Read the model definition and answer for the solid it produces. Units are mm, in the model's axes. Face numbers are marked on the shaded views. A direction names the side the tool comes from. Coordinates: 2 decimals unless noted, no trailing zeros. Write each loop counter-clockwise with the first axis right and the second up, starting at its lowest first coordinate (ties: lowest second). Pieces come first, ordered by that corner, then holes.
(1) Section B-B on y = 6.25 is taken. State how many separate pieces and enclosed holes the cut face has, then the cut area to 3 significant figures.
(2) Which of the six approach directions +Z, -Z, +X, -X, +Y, -Y give full straight-line access (tool end or side, diameter ignored) to the marked faces 4 and 5?
(3) Section A-A on x = 0 is taken. Write down the section's boundary in (y, z) (3 decimals), then the cut area to 3 significant figures.
(4) Given pin 1 (4 mm diameter, centred on x = -14, y = 3, fed in from -Z); pin 2 (6.5 mm diameter, centred on y = -1, z = 35, fed in from -X); pin 3 (11 mm diameter, centred on x = -43, y = -5, fed in from -Z); pin 4 (12 mm diameter, centred on x = -14, z = 55, fed in from +Y), each flat-ended and moving along its own axis, determine where each tip first touches the part or whether it passes through.
(5) Find the intervals of material crossed by probe 1 along Z at (x, y) = (-25.5, -3.5); probe 2 along X at (y, z) = (11.25, -43); probe 3 along X at (y, z) = (-9.75, -43), in increasing order.
(6) The mould has two halves that part along X. Classify the marked faces 1, 2 and 3: +X half, -X half, draft (parallel to the pull), parting line (faces both ways), or undercut.
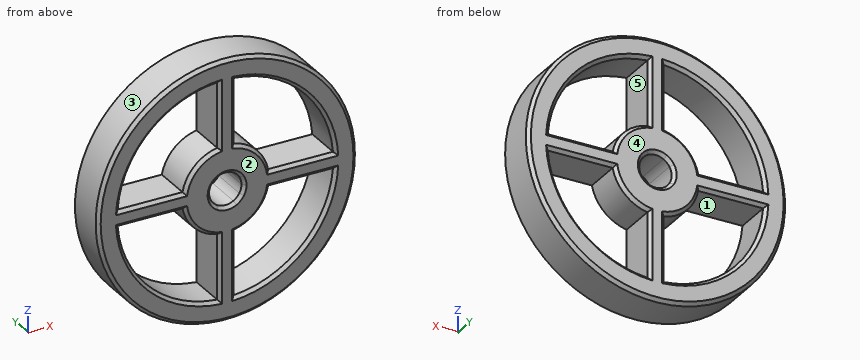
from build123d import *

# Parameters (mm, degrees)
F0_R     = 76.2
F1_DEPTH = 12.7
F2_SIZE  = 1.905
F3_SIZE  = 1.905


with BuildPart() as f1:
    # F0 (on Front) → F1 (new body, symmetric)
    with BuildSketch(Plane.XZ):
        Circle(F0_R)
        with BuildLine():
            ThreePointArc((-4.7625, -63.321154), (-44.901281, -44.901281), (-63.321154, -4.7625))
            Line((-63.321154, -4.7625), (-25.160792, -4.7625))
            Line((-25.160792, -4.7625), (-8.248892, -4.7625))
            ThreePointArc((-8.248892, -4.7625), (-9.525, 0), (-8.248892, 4.7625))
            Line((-8.248892, 4.7625), (-25.160792, 4.7625))
            Line((-25.160792, 4.7625), (-63.321154, 4.7625))
            ThreePointArc((-63.321154, 4.7625), (-44.901281, 44.901281), (-4.7625, 63.321154))
            Line((-4.7625, 63.321154), (-4.7625, 25.160792))
            Line((-4.7625, 25.160792), (-4.7625, 8.248892))
            ThreePointArc((-4.7625, 8.248892), (0, 9.525), (4.7625, 8.248892))
            Line((4.7625, 8.248892), (4.7625, 25.160792))
            Line((4.7625, 25.160792), (4.7625, 63.321154))
            ThreePointArc((4.7625, 63.321154), (44.901281, 44.901281), (63.321154, 4.7625))
            Line((63.321154, 4.7625), (25.160792, 4.7625))
            Line((25.160792, 4.7625), (8.248892, 4.7625))
            ThreePointArc((8.248892, 4.7625), (9.200443, 2.465251), (9.525, 0))
            ThreePointArc((9.525, 0), (9.200443, -2.465251), (8.248892, -4.7625))
            Line((8.248892, -4.7625), (25.160792, -4.7625))
            Line((25.160792, -4.7625), (63.321154, -4.7625))
            ThreePointArc((63.321154, -4.7625), (44.901281, -44.901281), (4.7625, -63.321154))
            Line((4.7625, -63.321154), (4.7625, -25.160792))
            Line((4.7625, -25.160792), (4.7625, -8.248892))
            ThreePointArc((4.7625, -8.248892), (0, -9.525), (-4.7625, -8.248892))
            Line((-4.7625, -8.248892), (-4.7625, -25.160792))
            Line((-4.7625, -25.160792), (-4.7625, -63.321154))
        make_face(mode=Mode.SUBTRACT)
        with BuildLine():
            Line((-25.160792, 4.7625), (-8.248892, 4.7625))
            ThreePointArc((-8.248892, 4.7625), (-6.735192, 6.735192), (-4.7625, 8.248892))
            Line((-4.7625, 8.248892), (-4.7625, 25.160792))
            ThreePointArc((-4.7625, 25.160792), (-18.107275, 18.107275), (-25.160792, 4.7625))
        make_face()
        with BuildLine():
            Line((4.7625, 25.160792), (4.7625, 8.248892))
            ThreePointArc((4.7625, 8.248892), (6.735192, 6.735192), (8.248892, 4.7625))
            Line((8.248892, 4.7625), (25.160792, 4.7625))
            ThreePointArc((25.160792, 4.7625), (18.107275, 18.107275), (4.7625, 25.160792))
        make_face()
        with BuildLine():
            ThreePointArc((8.248892, -4.7625), (6.735192, -6.735192), (4.7625, -8.248892))
            Line((4.7625, -8.248892), (4.7625, -25.160792))
            ThreePointArc((4.7625, -25.160792), (18.107275, -18.107275), (25.160792, -4.7625))
            Line((25.160792, -4.7625), (8.248892, -4.7625))
        make_face()
        with BuildLine():
            Line((-8.248892, -4.7625), (-25.160792, -4.7625))
            ThreePointArc((-25.160792, -4.7625), (-18.107275, -18.107275), (-4.7625, -25.160792))
            Line((-4.7625, -25.160792), (-4.7625, -8.248892))
            ThreePointArc((-4.7625, -8.248892), (-6.735192, -6.735192), (-8.248892, -4.7625))
        make_face()
    extrude(amount=F1_DEPTH, both=True)

    # F2
    f2_edges = [f1.edges().sort_by_distance(p)[0] for p in [
        (-76.2, -12.7, 0),
        (-4.7625, -12.7, -44.240973),
        (-44.901281, -12.7, -44.901281),
        (-44.240973, -12.7, -4.7625),
        (-18.107275, -12.7, -18.107275),
        (4.7625, -12.7, 8.248892),
        (44.240973, -12.7, -4.7625),
        (44.901281, -12.7, -44.901281),
        (4.7625, -12.7, -44.240973),
        (18.107275, -12.7, -18.107275),
        (4.7625, -12.7, 44.240973),
        (44.901281, -12.7, 44.901281),
        (44.240973, -12.7, 4.7625),
        (18.107275, -12.7, 18.107275),
        (-44.240973, -12.7, 4.7625),
        (-44.901281, -12.7, 44.901281),
        (-4.7625, -12.7, 44.240973),
        (-18.107275, -12.7, 18.107275),
    ]]
    chamfer(f2_edges, length=F2_SIZE)

    # F3
    f3_edges = [f1.edges().sort_by_distance(p)[0] for p in [
        (-76.2, 12.7, 0),
        (4.7625, 12.7, 8.248892),
        (-4.7625, 12.7, -44.240973),
        (-44.901281, 12.7, -44.901281),
        (-44.240973, 12.7, -4.7625),
        (-18.107275, 12.7, -18.107275),
        (44.240973, 12.7, -4.7625),
        (44.901281, 12.7, -44.901281),
        (4.7625, 12.7, -44.240973),
        (18.107275, 12.7, -18.107275),
        (4.7625, 12.7, 44.240973),
        (44.901281, 12.7, 44.901281),
        (44.240973, 12.7, 4.7625),
        (18.107275, 12.7, 18.107275),
        (-44.240973, 12.7, 4.7625),
        (-44.901281, 12.7, 44.901281),
        (-4.7625, 12.7, 44.240973),
        (-18.107275, 12.7, 18.107275),
    ]]
    chamfer(f3_edges, length=F3_SIZE)


solid = f1.part
Response:
1. separate pieces: 1
1. enclosed holes: 5
1. area: 8,800 mm2
2. face 4: +Z, -Z, +X, -X, +Y
2. face 5: +Y, -Y
3. outline: (-12.7, -74.295) - (-10.795, -76.2) - (10.795, -76.2) - (12.7, -74.295) - (12.7, -11.43) - (10.795, -9.525) - (-10.795, -9.525) - (-12.7, -11.43) - close; (-12.7, 11.43) - (-10.795, 9.525) - (10.795, 9.525) - (12.7, 11.43) - (12.7, 74.295) - (10.795, 76.2) - (-10.795, 76.2) - (-12.7, 74.295) - close
3. area: 3,370 mm2
4. pin 1: stops at z = -75.25
4. pin 2: stops at x = -69.27
4. pin 3: stops at z = -66.33
4. pin 4: passes through
5. probe 1: z = -71.81 to -58.15, -4.76 to 4.76, 58.15 to 71.81
5. probe 2: x = -62.36 to -47.34, -4.31 to 4.31, 47.34 to 62.36
5. probe 3: x = -62.91 to -46.73, -4.76 to 4.76, 46.73 to 62.91
6. face 1: undercut
6. face 2: draft
6. face 3: parting line
